Source: CAD feature listing. Evaluate the final solid. Frame: model axes, mm. A direction names the side the tool comes from. Coordinates: 2 decimals unless noted, no trailing zeros. Loops run counter-clockwise (first coordinate to the right, second up) from the corner with the lowest first, then second, coordinate; pieces in that order, holes last.
from build123d import *

# Parameters (mm, degrees)
SKETCH1_W           = 19.05
SKETCH1_H           = 5.7658
SKETCH1_H_2         = 5.5245
SKETCH1_H_3         = 5.461
SKETCH1_W_2         = 15.748
SKETCH1_H_4         = 20.828
SKETCH1_W_3         = 15.494
SKETCH1_H_5         = 20.574
SKETCH1_W_4         = 16.002
SKETCH1_H_6         = 21.082
SKETCH1_W_5         = 15.875
SKETCH1_H_7         = 20.955
SKETCH1_H_8         = 5.588
SKETCH1_H_9         = 5.715
SKETCH1_H_10        = 5.6642
BOSS_EXTRUDE1_DEPTH = 2.54


with BuildPart() as part:
    # Sketch1 → Boss-Extrude1 (new body)
    with BuildSketch(Plane(origin=(0, 0, 0), x_dir=(1, 0, 0), z_dir=(0, 1, 0))):
        Polygon((56.951560312, 84.213691439), (56.951560312, 75.188096428), (79.306647339, 75.188096428), (79.306647339, 71.525938437), (98.864647339, 71.525938437), (98.864647339, 75.188096428), (153.617936559, 75.188096428), (153.617936559, 86.784930064), (157.585274382, 86.784930064), (157.585274382, 106.165130064), (153.617936559, 106.165130064), (153.617936559, 141.820891439), (121.062786422, 141.820891439), (121.062786422, 145.967343453), (101.631786422, 145.967343453), (101.631786422, 141.820891439), (56.951560312, 141.820891439), (56.951560312, 134.591745655), (56.953910325, 134.591745655), (56.953910325, 116.049745655), (56.951560312, 116.049745655), (56.951560312, 103.720891439), (53.296575292, 103.720891439), (53.296575292, 84.213691439), align=None)
        with Locations((75.457604332, 115.587849021)):
            Rectangle(SKETCH1_W, SKETCH1_H, mode=Mode.SUBTRACT)
        with Locations((138.957604332, 115.708499021)):
            Rectangle(SKETCH1_W, SKETCH1_H_2, mode=Mode.SUBTRACT)
        with Locations((107.207604332, 115.740249021)):
            Rectangle(SKETCH1_W, SKETCH1_H_3, mode=Mode.SUBTRACT)
        with Locations((71.358442331, 95.058042907)):
            Rectangle(SKETCH1_W_2, SKETCH1_H_4, mode=Mode.SUBTRACT)
        with Locations((91.888312798, 94.844972613)):
            Rectangle(SKETCH1_W_3, SKETCH1_H_5, mode=Mode.SUBTRACT)
        with Locations((113.229534733, 95.098972613)):
            Rectangle(SKETCH1_W_4, SKETCH1_H_6, mode=Mode.SUBTRACT)
        with Locations((133.995045787, 95.035472613)):
            Rectangle(SKETCH1_W_5, SKETCH1_H_7, mode=Mode.SUBTRACT)
        with Locations((75.70300706, 129.926754737)):
            Rectangle(SKETCH1_W, SKETCH1_H_8, mode=Mode.SUBTRACT)
        with Locations((139.20300706, 129.863254737)):
            Rectangle(SKETCH1_W, SKETCH1_H_9, mode=Mode.SUBTRACT)
        with Locations((107.45300706, 129.888654737)):
            Rectangle(SKETCH1_W, SKETCH1_H_10, mode=Mode.SUBTRACT)
    extrude(amount=BOSS_EXTRUDE1_DEPTH)


solid = part.part
Q1. Access query for faces 4 (the flat face through (138, 1, -141.821)), 5 (the flat face through (105, 0, -109)), 6 (the flat face through (79.232, 1, -95)), 7 (the flat face through (56.954, 1, -125)). Directions: +Z, -Z, +X, -X, +Y, -Y. A direction counts if a zero-diameter tool reaches every point of the face in a straight line with its end or side. Return the directions, or none.
Q2. Line query: line 1 along Z through (x, y) = (82.5, 1.9); line 2 along X through (y, z) = (1.65, -113.5); line 3 along Z through (x, y) = (72, 1.2). Output: solid intervals per line, ascending.
Q3. Contact query for flat-ended pins moving along their axis: pin 1 Ø0.8 at (y, z) = (1, -116) entering from -X; pin 2 Ø1 at (x, y) = (86.5, 1) entering from -Z; pin 3 Ø1.5 at (x, y) = (114, 2) entering from +Z. Output: stop coordinate, or through.
Q4. Draft query along Z for faces 1 (the flat face through (99.635, 1, -95)), 2 (the flat face through (68, 1, -75.188)), 3 (the flat face through (121.063, 1, -144)). Return one class per face: +Z half, -Z half, draft (parallel to the pull), parting line (faces both ways), or undercut.
Q5. Section D-D, the plane x = 77.5. Return the cut outline in (y, z), plus the area to 3 significant figures.
Q6. Section A-A, the plane x = 91.5. Return the cut outline in (y, z).
Q7. Section C-C, the plane x = 136. Return the cut outline in (y, z), plus the area to 3 significant figures.
Q8. Section B-B, the plane z = -90.5. Return the cut outline in (x, y), plus the area to 3 significant figures.
Derived:
1. face 4: -Z, +X, +Y, -Y
1. face 5: +Z, -Z, +X, -X, -Y
1. face 6: +Y, -Y
1. face 7: -Z, -X, +Y, -Y
2. line 1: z = -141.82 to -132.72, -127.13 to -118.47, -112.7 to -71.53
2. line 2: x = 56.95 to 65.93, 84.98 to 97.68, 116.73 to 129.43, 148.48 to 153.62
2. line 3: z = -141.82 to -132.72, -127.13 to -118.47, -112.7 to -105.47, -84.64 to -75.19
3. pin 1: stops at x = 56.95
3. pin 2: stops at z = -141.82
3. pin 3: stops at z = -75.19
4. face 1: undercut
4. face 2: +Z half
4. face 3: draft
5. outline: (0, -141.82) - (2.54, -141.82) - (2.54, -132.72) - (0, -132.72) - close; (0, -127.13) - (2.54, -127.13) - (2.54, -118.47) - (0, -118.47) - close; (0, -112.7) - (2.54, -112.7) - (2.54, -105.47) - (0, -105.47) - close; (0, -84.64) - (2.54, -84.64) - (2.54, -75.19) - (0, -75.19) - close
5. area: 87.5 mm2
6. outline: (0, -141.82) - (2.54, -141.82) - (2.54, -105.13) - (0, -105.13) - close; (0, -84.56) - (2.54, -84.56) - (2.54, -71.53) - (0, -71.53) - close
7. outline: (0, -141.82) - (2.54, -141.82) - (2.54, -132.72) - (0, -132.72) - close; (0, -127.01) - (2.54, -127.01) - (2.54, -118.47) - (0, -118.47) - close; (0, -112.95) - (2.54, -112.95) - (2.54, -105.51) - (0, -105.51) - close; (0, -84.56) - (2.54, -84.56) - (2.54, -75.19) - (0, -75.19) - close
7. area: 87.5 mm2
8. outline: (53.3, 0) - (63.48, 0) - (63.48, 2.54) - (53.3, 2.54) - close; (79.23, 0) - (84.14, 0) - (84.14, 2.54) - (79.23, 2.54) - close; (99.64, 0) - (105.23, 0) - (105.23, 2.54) - (99.64, 2.54) - close; (121.23, 0) - (126.06, 0) - (126.06, 2.54) - (121.23, 2.54) - close; (141.93, 0) - (157.59, 0) - (157.59, 2.54) - (141.93, 2.54) - close
8. area: 105 mm2
